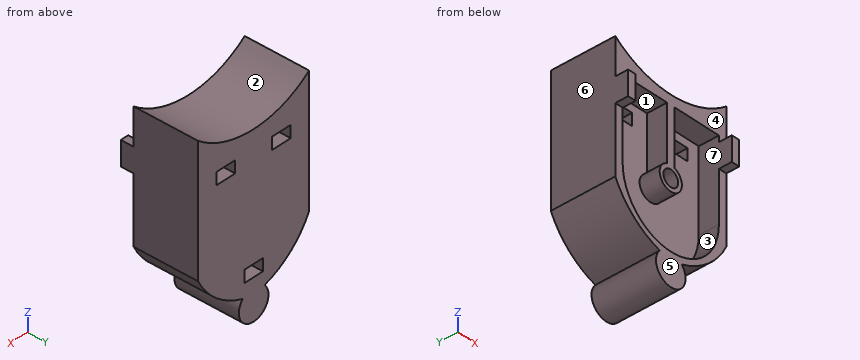
Autodesk Inventor part; units mm, degrees
ref_plane "YZ Plane" through (0, 0, 0) normal (1, 0, 0) x (0, 1, 0)
ref_plane "XZ Plane" through (0, 0, 0) normal (0, 1, 0) x (-1, 0, 0)
ref_plane "XY Plane" through (0, 0, 0) normal (0, 0, 1) x (1, 0, 0)
sketch "Sketch1" plane through (0, 0, 0) normal (0, 1, 0) x (-1, 0, 0)
  line L0 (-7.5, 5.5) -> (7.5, 5.5)
  line L1 (7.5, 5.5) -> (7.5, -5.5)
  line L2 (7.5, -5.5) -> (-7.5, -5.5)
  line L3 (-7.5, -5.5) -> (-7.5, 5.5)
  line L4 (-7.5, 5.5) -> (7.5, -5.5) construction
  line L5 (7.5, 5.5) -> (-7.5, -5.5) construction
  circle A0 centre (0, -5.5) radius 7.5 construction
  arc A1 (-7.5, -5.5) -> (7.5, -5.5) centre (0, -5.5) ccw
  point P0 (0, 0)
  dimension "d0" = 11
  dimension "d1" = 15
extrude "Extrusion1" add sketch "Sketch1" along normal blind 8
sketch "Sketch2" plane through (0, 0, 0) normal (0, -1, 0) x (1, 0, 0)
  line L0 (7.5, 9.25) -> (-7.5, 9.25)
  line L1 (-7.5, 9.25) -> (-7.5, -20.75)
  line L2 (-7.5, -20.75) -> (7.5, -20.75)
  line L3 (7.5, -20.75) -> (7.5, 9.25)
  line L4 (7.5, 9.25) -> (-7.5, -20.75) construction
  line L5 (-7.5, 9.25) -> (7.5, -20.75) construction
  line L6 (-7.5, 5.5) -> (7.5, 5.5)
  line L7 (7, 8.75) -> (-7, 8.75) construction
  line L8 (-7, 8.75) -> (-7, -20.25) construction
  line L9 (-7, -20.25) -> (7, -20.25) construction
  line L10 (7, -20.25) -> (7, 8.75) construction
  line L11 (7, 8.75) -> (-7, -20.25) construction
  line L12 (-7, 8.75) -> (7, -20.25) construction
  point P0 (0, 0)
  point P1 (0, -5.75)
  dimension "d4" = 15
  dimension "d5" = 30
  dimension "d6" = 3.75
  dimension "d18" = 0.5
  dimension "d19" = 0.5
sketch "Sketch4" plane through (0, 0, 0) normal (0, -1, 0) x (1, 0, 0)
  line L0 (-7.5, -5.5) -> (-7.5, 5.5)
  line L1 (-7.5, 3.75) -> (-6.5, 3.75)
  line L2 (-6.5, 3.75) -> (-6.5, 0.75)
  line L3 (-6.5, 0.75) -> (-7.5, 0.75)
  line L4 (-7.5, 0.75) -> (-7.5, 3.75)
  line L5 (7.5, 5.5) -> (7.5, -5.5)
  line L6 (7.5, 0.75) -> (6.5, 0.75)
  line L7 (6.5, 0.75) -> (6.5, 3.75)
  line L8 (6.5, 3.75) -> (7.5, 3.75)
  line L9 (7.5, 3.75) -> (7.5, 0.75)
  line L10 (-7.5, -20.25) -> (7.5, -20.25) construction
  line L11 (7.5, -20.25) -> (7.5, 9.75) construction
  line L12 (7.5, 9.75) -> (-7.5, 9.75) construction
  line L13 (-7.5, 9.75) -> (-7.5, -20.25) construction
  line L14 (-7.5, -20.25) -> (7.5, 9.75) construction
  line L15 (7.5, -20.25) -> (-7.5, 9.75) construction
  line L16 (-7.5, 5.5) -> (7.5, 5.5) construction
  arc A0 (-7.5, -5.5) -> (7.5, -5.5) centre (0, -5.5) ccw construction
  point P0 (0, 0)
  point P1 (0, -5.25)
  point P2 (0, -13)
  point P3 (-7, 3.75)
  point P4 (-7.5, 0.75)
  point P5 (-7, 0.75)
  point P6 (7.5, 3.75)
  point P7 (-7.5, 0.75)
  dimension "d20" = 1
  dimension "d21" = 3
  dimension "d22" = 1
  dimension "d23" = 3
  dimension "d24" = 15
  dimension "d25" = 30
  dimension "d27" = 7.25
  dimension "d106" = 0.75
extrude "Extrusion3" add sketch "Sketch4" along normal blind 1.6
sketch "Sketch6" plane through (0, 0, 0) normal (0, -1, 0) x (1, 0, 0)
  line L0 (7.5, 11.25) -> (-7.5, 11.25)
  line L1 (-7.5, 11.25) -> (-7.5, -18.75)
  line L2 (-7.5, -18.75) -> (7.5, -18.75)
  line L3 (7.5, -18.75) -> (7.5, 11.25)
  line L4 (7.5, 11.25) -> (-7.5, -18.75) construction
  line L5 (-7.5, 11.25) -> (7.5, -18.75) construction
  line L6 (7, 10.75) -> (-7, 10.75) construction
  line L7 (-7, 10.75) -> (-7, -18.25) construction
  line L8 (-7, -18.25) -> (7, -18.25) construction
  line L9 (7, -18.25) -> (7, 10.75) construction
  line L10 (7, 10.75) -> (-7, -18.25) construction
  line L11 (-7, 10.75) -> (7, -18.25) construction
  circle A0 centre (0, -3.75) radius 1
  circle A1 centre (0, -3.75) radius 1.5
  line L12 (-6.5, 4.5) -> (6.5, 4.5)
  line L13 (6.5, 4.5) -> (6.5, -5.5)
  line L14 (6.5, -5.5) -> (-6.5, -5.5)
  line L15 (-6.5, -5.5) -> (-6.5, 4.5)
  line L16 (-7.5, 5.5) -> (7.5, 5.5)
  arc A2 (-7.5, -5.5) -> (7.5, -5.5) centre (0, -5.5) ccw
  circle A3 centre (0, -5.5) radius 6.5
  point P0 (0, 0)
  point P1 (-7.5, -3.75)
  point P2 (6.5, -5.5)
  dimension "d31" = 15
  dimension "d32" = 30
  dimension "d34" = 0.5
  dimension "d35" = 0.5
  dimension "d36" = 2
  dimension "d37" = 0.5
  dimension "d38" = 1
  dimension "d39" = 1
  dimension "d40" = 1
  dimension "d41" = 1
  dimension "d107" = 3.75
extrude "Extrusion4" cut sketch "Sketch6" against normal blind 2.5 contours A0 | L12 L13 A3 L15 | A3 L14 | L14 A3
sketch "Sketch10" plane through (0, 8, 0) normal (0, 1, 0) x (1, 0, 0)
  point P0 (0, 0)
sketch "Sketch11" plane through (0, 0, 0) normal (0, -1, 0) x (1, 0, 0)
  line L0 (-5, 3.5) -> (-2.5, 3.5)
  line L1 (-2.5, 3.5) -> (-2.5, 2)
  line L2 (-2.5, 2) -> (-5, 2)
  line L3 (-5, 2) -> (-5, 3.5)
  line L4 (2.5, 3.5) -> (5, 3.5)
  line L5 (5, 3.5) -> (5, 2)
  line L6 (5, 2) -> (2.5, 2)
  line L7 (2.5, 2) -> (2.5, 3.5)
  line L8 (-6.5, 3.75) -> (-7.5, 3.75)
  line L9 (-6.5, 0.75) -> (-6.5, 3.75)
  line L10 (6.5, 3.75) -> (6.5, 0.75)
  line L11 (-6.5, 4.5) -> (6.5, 4.5)
  line L12 (-1.25, -11) -> (1.25, -11)
  line L13 (1.25, -11) -> (1.25, -9.5)
  line L14 (1.25, -9.5) -> (-1.25, -9.5)
  line L15 (-1.25, -9.5) -> (-1.25, -11)
  circle A0 centre (0, -3.75) radius 1
  point P0 (0, 0)
  point P1 (-3.75, 3.5)
  point P2 (3.75, 3.5)
  point P3 (1.25, -10.25)
  point P4 (2.5, 2.75)
  point P5 (0, -9.5)
  point P6 (3.75, 2)
  point P7 (-2.5, 2.75)
  dimension "d51" = 2.5
  dimension "d52" = 1.5
  dimension "d55" = 2.75
  dimension "d56" = 2.75
  dimension "d60" = 13
  dimension "d61" = 3.75
  dimension "d62" = 3.75
  dimension "d103" = 6.5
  dimension "d104" = 6.5
extrude "Extrusion8" cut sketch "Sketch11" against normal blind 10 contours L0 L1 L2 L3 | L4 L5 L6 L7 | L15 L14 L13 L12
sketch "Sketch12" plane through (0, 2.5, 0) normal (0, -1, 0) x (1, 0, 0)
  line L0 (5, 2) -> (5, 3.5) construction
  line L1 (2.5, 2) -> (5, 2) construction
  line L2 (5, 3.5) -> (2.5, 3.5) construction
  line L3 (2.5, 3.5) -> (2.5, 2) construction
  line L4 (2.5, 2) -> (5, 2) construction
  line L5 (5, 2) -> (5, 3.5) construction
  line L6 (-2.5, 2) -> (-2.5, 3.5) construction
  line L7 (-2.5, 2) -> (-5, 2) construction
  line L8 (-2.5, 3.5) -> (-5, 3.5) construction
  line L9 (-5, 3.5) -> (-5, 2) construction
  line L10 (-5, 2) -> (-2.5, 2) construction
  line L11 (-2.5, 2) -> (-2.5, 3.5) construction
  line L12 (-1.25, -9.5) -> (1.25, -9.5) construction
  line L13 (-1.25, -9.5) -> (-1.25, -11) construction
  line L14 (1.25, -9.5) -> (-1.25, -9.5) construction
  line L15 (-1.25, -9.5) -> (-1.25, -11) construction
  line L16 (-1.25, -11) -> (1.25, -11) construction
  line L17 (1.25, -11) -> (1.25, -9.5) construction
  line L18 (5.5, 3.5) -> (2, 3.5)
  line L19 (2, 3.5) -> (2, 2)
  line L20 (2, 2) -> (5.5, 2)
  line L21 (5.5, 2) -> (5.5, 3.5)
  line L22 (1.75, -9.5) -> (-1.75, -9.5)
  line L23 (-1.75, -9.5) -> (-1.75, -11)
  line L24 (-1.75, -11) -> (1.75, -11)
  line L25 (1.75, -11) -> (1.75, -9.5)
  line L26 (-2, 3.5) -> (-5.5, 3.5)
  line L27 (-5.5, 3.5) -> (-5.5, 2)
  line L28 (-5.5, 2) -> (-2, 2)
  line L29 (-2, 2) -> (-2, 3.5)
  point P0 (0, 0)
  point P1 (-2.5, 2.75)
  point P2 (-2, 2.75)
  point P3 (-3.75, 2)
  point P4 (-3.75, 2)
  point P5 (-3.75, 3.5)
  point P6 (-3.75, 3.5)
  point P7 (-5, 2.75)
  point P8 (-5.5, 2.75)
  point P9 (1.25, -10.25)
  point P10 (1.75, -10.25)
  point P11 (0, -11)
  point P12 (-1.25, -10.25)
  dimension "d63" = 0.5
  dimension "d64" = 0
  dimension "d65" = 0
  dimension "d67" = 0.5
  dimension "d68" = 0
  dimension "d69" = 0
  dimension "d70" = 0.5
  dimension "d71" = 0.5
  dimension "d72" = 0
  dimension "d73" = 0
  dimension "d74" = 0.5
  dimension "d96" = 0.5
sketch "Sketch16" plane through (0, 2.5, 0) normal (0, -1, 0) x (1, 0, 0)
  line L0 (-6.5, -5.5) -> (-6.5, 4.5) construction
  line L1 (-6.5, 4.5) -> (6.5, 4.5) construction
  line L2 (-6.5, 4.5) -> (6.5, 4.5) construction
  line L3 (-0.5, 4.5) -> (0.5, 4.5)
  line L4 (0.5, 4.5) -> (0.5, -2.75)
  line L5 (0.5, -2.75) -> (-0.5, -2.75)
  line L6 (-0.5, -2.75) -> (-0.5, 4.5)
  circle A0 centre (0, -3.75) radius 1.5 construction
  circle A1 centre (0, -3.75) radius 1.75 construction
  line L7 (-6.5, -2.75) -> (6.5174, -2.75) construction
  circle A2 centre (0, -3.75) radius 1.5 construction
  circle A3 centre (0, -3.75) radius 1 construction
  line L8 (6.5, 0.75) -> (6.5, -5.5)
  line L9 (-6.5, -5.873) -> (6.5, -5.873)
  line L10 (6.5, -5.873) -> (6.5, -6.873)
  line L11 (6.5, -6.873) -> (-6.5, -6.873)
  line L12 (-6.5, -6.873) -> (-6.5, -5.873)
  point P0 (0, 0)
  point P1 (0, 4.5)
  point P2 (0.0087, -2.75)
  dimension "d94" = 1
  dimension "d95" = 1
extrude "Extrusion10" add sketch "Sketch16" along normal blind 2.5 contours L3 L4 L5 L6
sketch "Sketch19" plane through (-7.5, 0, 5.5) normal (0, 0, 1) x (1, 0, 0)
  line L0 (15, 0) -> (15, 8)
  line L1 (0, 8) -> (15, 8)
  line L2 (15, 8) -> (15, 0)
  line L3 (15, 0) -> (0, 0)
  line L4 (0, 0) -> (0, 8)
  point P0 (7.5, 0)
extrude "Extrusion13" add sketch "Sketch19" along normal blind 6
sketch "Sketch18" plane through (0, 8, 0) normal (0, 1, 0) x (1, 0, 0)
  line L0 (-7.5, -3.75) -> (-7.5, -5.5)
  line L1 (-7.5, -5.5) -> (-7.5, -8.2917)
  line L2 (7.5, -5.5) -> (7.5, -8.2917)
  arc A0 (7.5, -8.2917) -> (-7.5, -8.2917) centre (0, -17.6592) ccw
  line L3 (-7.5, -5.5) -> (0, -3.75)
  line L4 (-7.5, -5.5) -> (7.5, -5.5)
  line L5 (0, -3.75) -> (7.5, -5.5)
  line L6 (-7.5, -8.2917) -> (-7.5, -17.8663)
  line L7 (-7.5, -17.8663) -> (8.2387, -17.8663)
  line L8 (8.2387, -17.8663) -> (7.5, -8.2917)
  line L9 (-7.5, -8.2917) -> (-7.5, -5.5)
  point P0 (0, 0)
  point P1 (3.395, -5.5)
  point P2 (-3.395, -5.5)
  dimension "d108" = 12
extrude "Extrusion12" cut sketch "Sketch18" against normal blind 8 contours A0 L8 L7 L6
sketch "Sketch21" plane through (0, 8, 0) normal (0, 1, 0) x (1, 0, 0)
  line L0 (-7.5, 5.5) -> (-7.5, -8.2917)
  line L1 (-7.5, 5.5) -> (-4.5586, 5.5)
  line L2 (-4.5586, 5.5) -> (-4.5586, 13.4633)
  line L3 (-4.5586, 13.4633) -> (-7.5, 13.4633)
  line L4 (-7.5, 13.4633) -> (-7.5, 5.5)
  arc A0 (7.5, 5.5) -> (-7.5, 5.5) centre (0, 5.5) ccw
  line L5 (7.5, 5.5) -> (3.8632, 5.5)
  line L6 (3.8632, 5.5) -> (3.8632, 13.1156)
  line L7 (3.8632, 13.1156) -> (7.5, 13.1156)
  line L8 (7.5, 13.1156) -> (7.5, 5.5)
  point P0 (0, 0)
  point P1 (3.8632, 11.9285)
  point P2 (-4.5586, 11.4556)
  point P3 (-7.5, -5.5)
extrude "Extrusion15" add sketch "Sketch21" against normal blind 8 contours L6 L7 L8 A0 | L4 L3 L2 A0
sketch "Sketch20" plane through (0, 8, 0) normal (0, 1, 0) x (1, 0, 0)
  arc A0 (7.5, 5.5) -> (-7.5, 5.5) centre (0, 5.5) ccw
  line L0 (-7.5, 5.5) -> (-7.5, 7.5)
  line L1 (7.5, 5.5) -> (7.5, 7.5)
  arc A1 (0, 13) -> (-7.5, 7.5) centre (1.4853, 3.1109) ccw
  arc A2 (7.5, 7.5) -> (0, 13) centre (-1.4853, 3.1109) ccw
  line L2 (-7.5, 7.5) -> (-7.5, 19.3065)
  line L3 (-7.5, 7.5) -> (4.3065, 7.5) construction
  line L4 (-7.5, 19.3065) -> (7.5, 19.3065)
  line L5 (7.5, 19.3065) -> (7.5, 7.5)
  point P0 (0, 0)
  point P1 (-6.7259, 8.8184)
  point P2 (6.7259, 8.8184)
  dimension "d113" = 2
  dimension "d114" = 10
  dimension "d115" = 90
  dimension "d116" = 90
extrude "Extrusion14" cut sketch "Sketch20" against normal blind 10 contours A2 A0 | A0 A1 L2 L4 L5 A2 | A1 A0
sketch "Sketch22" plane through (0, 8, 0) normal (0, 1, 0) x (1, 0, 0)
  line L0 (0, 0) -> (0, 20.304) construction
  circle A0 centre (0, 14) radius 2
  line L1 (-1.25, 11) -> (1.25, 11)
  dimension "d121" = 4
  dimension "d122" = 3
extrude "Extrusion16" add sketch "Sketch22" against normal blind 8
sketch "Sketch23" plane through (0, 2.5, -3.75) normal (0, -1, 0) x (1, 0, 0)
  circle A0 centre (0, 0) radius 1
  circle A1 centre (0, 0) radius 1
  point P0 (0, 3.75)
extrude "Extrusion17" cut sketch "Sketch23" against normal blind 3
sketch "Sketch14" plane through (0, 2.5, 0) normal (0, -1, 0) x (1, 0, 0)
  line L0 (5, 2.75) -> (2.5, 2.75) construction
  line L1 (2.5, 2.75) -> (2.5, 1.25) construction
  line L2 (2.5, 1.25) -> (5, 1.25) construction
  line L3 (5, 1.25) -> (5, 2.75) construction
  line L4 (5.5, 3.25) -> (2, 3.25)
  line L5 (2, 3.25) -> (2, 0.75)
  line L6 (2, 0.75) -> (5.5, 0.75)
  line L7 (5.5, 0.75) -> (5.5, 3.25)
  dimension "d86" = 0.5
  dimension "d87" = 0.5
sketch "Sketch15" plane through (0, 3.5, 0) normal (0, -1, 0) x (1, 0, 0)
  line L0 (5, 2.75) -> (2.5, 2.75)
  line L1 (2.5, 2.75) -> (2.5, 1.25)
  line L2 (2.5, 1.25) -> (5, 1.25)
  line L3 (5, 1.25) -> (5, 2.75)
  point P0 (0, 0)
sketch "Sketch8" plane through (0, 0, -3.75) normal (0, -1, 0) x (1, 0, 0)
  circle A0 centre (0, 0) radius 1.75
  circle A1 centre (0, 0) radius 1.5
  circle A2 centre (0, 0) radius 1.5
  point P0 (0, 3.75)
  dimension "d46" = 0.25
sketch "Sketch7" plane through (0, 2.5, -3.75) normal (0, -1, 0) x (1, 0, 0)
  circle A0 centre (0, 0) radius 1.25
  point P0 (0, 3.75)
properties part number "NORGATE"
Geometry: final body of the model. Coordinates: model frame, mm. Face numbers are marked on the shaded views. A direction names the side the tool comes from. Round coordinates to 2 decimals unless told otherwise and drop trailing zeros. Order: outer loops, then holes, each group sorted by start corner. A loop starts at its lowest first (then second) coordinate and runs counter-clockwise, first axis right, second up. Notation, with made-up numbers: (70, 23.25) -> (93, 23.25) arc R18 ccw to (93, 38.25) -> close; hole circle Ø10 at (47.25, -34). An arc over 180 degrees is marked (long way). Write each question's results on one line, items separated by ' | '.
Q1. Pull-direction query (Z, two-part tool) for the marked faces 1, 2, 3 and 4; classes: released by +Z, released by -Z, zero draft, split by the parting line, or undercut.
Response values:
face 1: undercut | face 2: released by +Z | face 3: undercut | face 4: zero draft
Q2. Section query B-B (x = 0). Output: boundary loops of the cut face in (y, z), and give its area (3 significant figures).
Response values:
outline: (0, -16) -> (8, -16) -> (8, -11) -> (2.5, -11) -> (2.5, -12) -> (0, -12) -> close; (0, -5.25) -> (2.5, -5.25) -> (2.5, -9.5) -> (8, -9.5) -> (8, 5.66) -> (0, 5.66) -> (0, -2.75) -> (5.5, -2.75) -> (5.5, -4.75) -> (0, -4.75) -> close | area: 137 mm²
Q3. Section query C-C (y = 4.75). Output: boundary loops of the cut face in (x, z).
Response values:
outline: (-7.5, -7.5) arc R10 ccw to (-1.48, -12.66) arc R2 ccw (long way) to (1.48, -12.66) arc R10 ccw to (7.5, -7.5) -> (7.5, 8.29) arc R12 cw to (-7.5, 8.29) -> close; hole (-5, 2) -> (-2.5, 2) -> (-2.5, 3.5) -> (-5, 3.5) -> close; hole (-1.25, -11) -> (1.25, -11) -> (1.25, -9.5) -> (-1.25, -9.5) -> close; hole circle Ø2 at (0, -3.75); hole (2.5, 2) -> (5, 2) -> (5, 3.5) -> (2.5, 3.5) -> close
Q4. Section query A-A (y = -0.75). Output: boundary loops of the cut face in (x, z).
Response values:
outline: (-7.5, 0.75) -> (-6.5, 0.75) -> (-6.5, 3.75) -> (-7.5, 3.75) -> close; (6.5, 0.75) -> (7.5, 0.75) -> (7.5, 3.75) -> (6.5, 3.75) -> close
Q5. Access query for the marked faces 5, 6 and 7. Directions: +Z, -Z, +X, -X, +Y, -Y. A direction counts if a zero-diameter tool reaches every point of the face in a straight line with its end or side. Return the directions, or none.
Response values:
face 5: -Z, +X, -X, -Y | face 6: +Z, -Z, -X, +Y, -Y | face 7: -Y
Q6. Ray query, line 1 along Z through (x, y) = (0, 3.7); line 2 along X through (y, z) = (4.3, -3.75); line 3 along Y through (x, z) = (-5, -2.5). Return the intervals inside material, ascending.
Response values:
line 1: -16 to -11, -9.5 to -4.75, -2.75 to 5.66 | line 2: -7.5 to -1, 1 to 7.5 | line 3: 2.5 to 8
Q7. Section query D-D (z = 2.5). Output: boundary loops of the cut face in (x, y).
Response values:
outline: (-7.5, -1.6) -> (-6.5, -1.6) -> (-6.5, 2.5) -> (-5, 2.5) -> (-5, 8) -> (-7.5, 8) -> close; (-2.5, 2.5) -> (-0.5, 2.5) -> (-0.5, 0) -> (0.5, 0) -> (0.5, 2.5) -> (2.5, 2.5) -> (2.5, 8) -> (-2.5, 8) -> close; (5, 2.5) -> (6.5, 2.5) -> (6.5, -1.6) -> (7.5, -1.6) -> (7.5, 8) -> (5, 8) -> close
Q8. Pin query (flat end, axial travel): pin 1 Ø1 at (x, y) = (-5, 5) entering from +Z; pin 2 Ø2 at (x, y) = (-2, 2.5) entering from +Z; pin 3 Ø2 at (x, z) = (-0.5, -3.5) entering from -Y. Return the tip coordinate at first contact, or that it passes through.
Response values:
pin 1: z = 6.99 | pin 2: z = 6.04 | pin 3: y = 0
